```python
from build123d import *

# Parameters (mm, degrees)
SKETCH_1_R          = 1.5
EXTRUDE_1_DEPTH     = 1
SKETCH_2_R          = 2
SKETCH_2_W          = 15
SKETCH_2_H          = 20
CUT_EXTRUDE_1_DEPTH = 315.198981539
SKETCH_3_W          = 130
SKETCH_3_H          = 76
CUT_EXTRUDE_2_DEPTH = 315.198981539


with BuildPart() as part:
    # 草图1 → 凸台-拉伸1 (new body)
    with BuildSketch(Plane.XY):
        Polygon((0, 0), (0, 76), (25, 76), (25, 116), (267, 116), (267, 76), (292, 76), (292, 0), align=None)
        with Locations((3, 48)):
            Circle(SKETCH_1_R, mode=Mode.SUBTRACT)
        with Locations((3, 28)):
            Circle(SKETCH_1_R, mode=Mode.SUBTRACT)
        with Locations(Location((289, 28, 0), (0, 0, 180))):
            Circle(SKETCH_1_R, mode=Mode.SUBTRACT)
        with Locations(Location((289, 48, 0), (0, 0, 180))):
            Circle(SKETCH_1_R, mode=Mode.SUBTRACT)
    extrude(amount=EXTRUDE_1_DEPTH)

    # 草图2 → 切除-拉伸1 (cut, through all)
    with BuildSketch(Plane.XY.offset(1)):
        with Locations((65, 111)):
            Circle(SKETCH_2_R)
        with Locations(Location((227, 111, 0), (0, 0, 180))):
            Circle(SKETCH_2_R)
        with Locations((146, 111)):
            Circle(SKETCH_2_R)
        with Locations((193.5, 106)):
            Rectangle(SKETCH_2_W, SKETCH_2_H)
        with Locations((98.5, 106)):
            Rectangle(SKETCH_2_W, SKETCH_2_H)
    extrude(amount=-CUT_EXTRUDE_1_DEPTH, mode=Mode.SUBTRACT)

    # 草图3 → 切除-拉伸2 (cut, through all)
    with BuildSketch(Plane.XY.offset(1)):
        with Locations((227, 38)):
            Rectangle(SKETCH_3_W, SKETCH_3_H)
    extrude(amount=-CUT_EXTRUDE_2_DEPTH, mode=Mode.SUBTRACT)


solid = part.part
```
Can you work these out from the model? Positions are in its coordinate system, mm. Round coordinates to 2 decimals unless told otherwise and drop trailing zeros. Loops run counter-clockwise (first coordinate to the right, second up) from the corner with the lowest first, then second, coordinate; pieces in that order, holes last.
Item 1: Please list where these lines run through material, in increasing order: L1, parallel to Y at x = 3, z = 0.4; L2, parallel to X at y = 107.5, z = 0.2; L3, parallel to Y at x = 227, z = 0.15.
Item 2: Suppose I cut it at C-C, the plane y = 79. Write out the boundary of the cut face in (x, z), then the cut area to 3 significant figures.
Item 3: Suppose I cut it at B-B, the plane y = 102.5. Write out the boundary of the cut face in (x, z).
Item 4: Suppose I cut it at D-D, the plane y = 55.5. Write out the boundary of the cut face in (x, z).
Item 5: Suppose I cut it at A-A, the plane z = 0.45. Write out the boundary of the cut face in (x, y), then the cut area to 3 significant figures.
Item 6: Will these pins go through, and if not, where does the flat tip stop? pin 1 Ø0.5 at (y, z) = (110.5, 0.5) entering from -X; pin 2 Ø0.5 at (x, z) = (11.5, 0.5) entering from +Y.
Reported:
1. L1: y = 0 to 26.5, 29.5 to 46.5, 49.5 to 76
1. L2: x = 25 to 91, 106 to 186, 201 to 267
1. L3: y = 76 to 109, 113 to 116
2. outline: (25, 0) - (267, 0) - (267, 1) - (25, 1) - close
2. area: 242 mm2
3. outline: (25, 0) - (91, 0) - (91, 1) - (25, 1) - close; (106, 0) - (186, 0) - (186, 1) - (106, 1) - close; (201, 0) - (267, 0) - (267, 1) - (201, 1) - close
4. outline: (0, 0) - (162, 0) - (162, 1) - (0, 1) - close
5. outline: (0, 0) - (162, 0) - (162, 76) - (267, 76) - (267, 116) - (201, 116) - (201, 96) - (186, 96) - (186, 116) - (106, 116) - (106, 96) - (91, 96) - (91, 116) - (25, 116) - (25, 76) - (0, 76) - close; hole circle Ø3 at (3, 28); hole circle Ø3 at (3, 48); hole circle Ø4 at (65, 111); hole circle Ø4 at (146, 111); hole circle Ø4 at (227, 111)
5. area: 21,300 mm2
6. pin 1: stops at x = 25
6. pin 2: stops at y = 76
